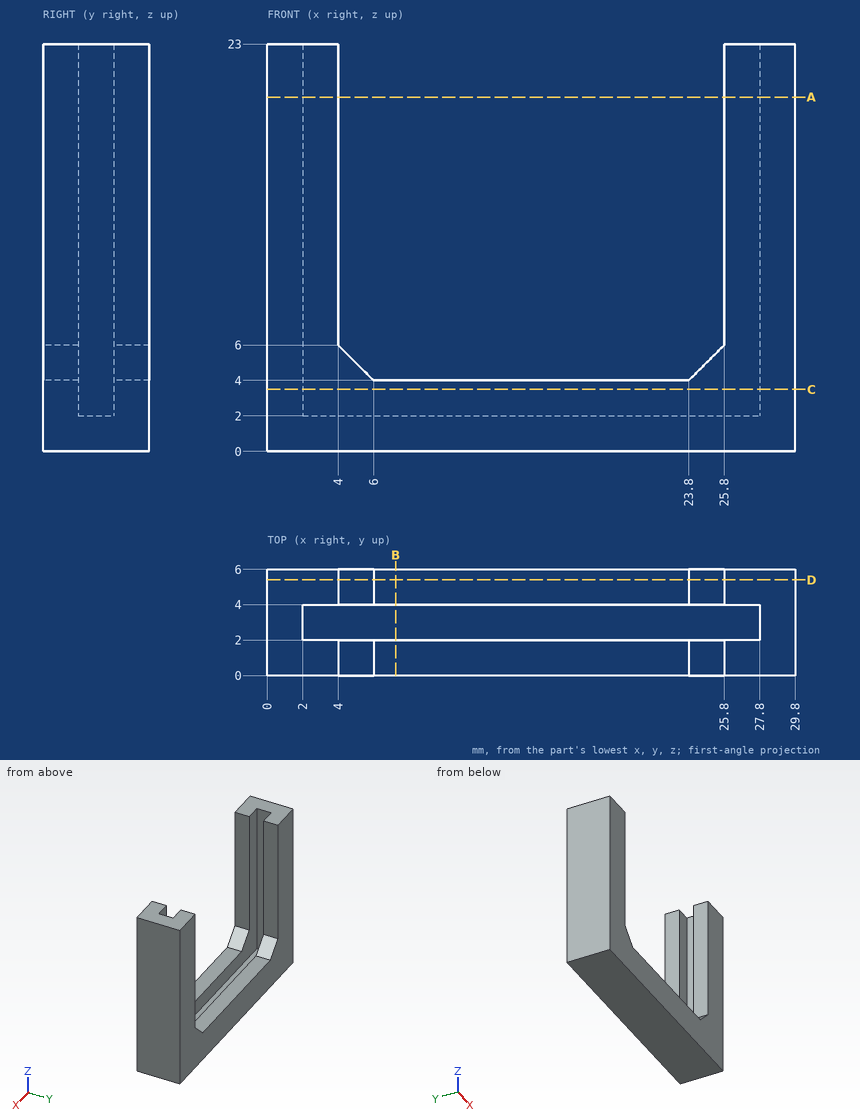
For this review, use the dimensioned drawing (mm, ordinates from the lowest corner) and the shaded views. Round coordinates to 2 decimals unless told otherwise and drop trailing zeros. Loops run counter-clockwise (first coordinate to the right, second up) from the corner with the lowest first, then second, coordinate; pieces in that order, holes last. Notation, with made-up numbers: M 0,71 L 30,71 A8 cw 30,86 Z; hole C 41,86.5 d9. An arc over 180 degrees is marked long. Answer as a JSON object with one key per item and string values.
(1) Clearance check with flat-ended pins moving along their axes: P1, Ø1, axis at x = 11, y = 3, coming from the +Z side; P2, Ø6.5, axis at x = 9, z = 15, coming from the +Y side; P3, Ø0.6, axis at x = 10.5, y = 5, coming from the +Z side. State where each tip first meets the part, or that it passes through.
Resolved:
{"P1": "z = 2", "P2": "through", "P3": "z = 4"}
(2) Take a section at C-C on z = 3.5. Give the boundary of the cut face in (x, y), and give its area (3 significant figures).
Resolved:
{"outline": "M 0,0 L 29.8,0 L 29.8,6 L 0,6 Z; hole M 2,2 L 27.8,2 L 27.8,4 L 2,4 Z", "area": "127 mm²"}
(3) Take a section at B-B on x = 7.25. Give the boundary of the cut face in (y, z).
Resolved:
{"outline": "M 0,0 L 6,0 L 6,4 L 4,4 L 4,2 L 2,2 L 2,4 L 0,4 Z"}
(4) To check wall thickness, follow line 1 along X through (y, z) = (3.4, 19.75); line 2 along Y through (x, z) = (27, 6.75); line 3 along X through (y, z) = (1.9, 9). State the ranges of each line that lie inside material, in increasing order.
Resolved:
{"line 1": "0 to 2, 27.8 to 29.8", "line 2": "0 to 2, 4 to 6", "line 3": "0 to 4, 25.8 to 29.8"}
(5) Take a section at A-A on z = 20. Give the boundary of the cut face in (x, y).
Resolved:
{"outline": "M 0,0 L 4,0 L 4,2 L 2,2 L 2,4 L 4,4 L 4,6 L 0,6 Z; M 25.8,0 L 29.8,0 L 29.8,6 L 25.8,6 L 25.8,4 L 27.8,4 L 27.8,2 L 25.8,2 Z"}
(6) Take a section at D-D on y = 5.4. Give the boundary of the cut face in (x, z), and give its area (3 significant figures).
Resolved:
{"outline": "M 0,0 L 29.8,0 L 29.8,23 L 25.8,23 L 25.8,6 L 23.8,4 L 6,4 L 4,6 L 4,23 L 0,23 Z", "area": "275 mm²"}
